Geometry: final body of the model. Coordinates: model frame, mm. A direction names the side the tool comes from. Coordinates: 2 decimals unless noted, no trailing zeros. Write each loop counter-clockwise with the first axis right and the second up, starting at its lowest first coordinate (ties: lowest second). Pieces come first, ordered by that corner, then holes. Notation, with made-up numbers: (-22, 35) -> (-17, 35) arc R36 ccw to (-17, 72) -> close; hole circle Ø6 at (-17, 72.5). An arc over 180 degrees is marked (long way). Answer as a JSON object with one key per item and string values. Group by question number.
```python
from build123d import *

# Parameters (mm, degrees)
SKETCH1_R             = 3
BOSS_EXTRUDE1_DEPTH   = 25
FILLET2_R             = 2
CUT_EXTRUDE1_DEPTH    = 26
M5_TAPPED_HOLE1_D     = 4.2
M5_TAPPED_HOLE1_DEPTH = 22.4
M5_TAPPED_HOLE1_TIP   = 1.2618073
M5_TAPPED_HOLE2_D     = 4.2
M5_TAPPED_HOLE2_DEPTH = 22.4
M5_TAPPED_HOLE2_TIP   = 1.2618073
M4_TAPPED_HOLE1_D     = 3.3
M4_TAPPED_HOLE1_DEPTH = 10.1
M4_TAPPED_HOLE1_TIP   = 0.991420021
CHAMFER1_SIZE         = 1


with BuildPart() as part:
    # Sketch1 → Boss-Extrude1 (new body)
    with BuildSketch(Plane(origin=(0, 0, 0), x_dir=(0, 0, -1), z_dir=(1, 0, 0))):
        with BuildLine():
            Line((-33.809460939, 72.504622963), (-30.428514845, 65.254160667))
            ThreePointArc((-30.428514845, 65.254160667), (-17.004346403, 64.269330845), (-4.58110934, 59.088465181))
            Line((-4.58110934, 59.088465181), (10.41889066, 59.088465181))
            Line((10.41889066, 59.088465181), (13.891854213, 78.784620241))
            ThreePointArc((13.891854213, 78.784620241), (-10.442095378, 79.31558891), (-33.809460939, 72.504622963))
        make_face()
        with Locations((0, 70)):
            Circle(SKETCH1_R, mode=Mode.SUBTRACT)
    extrude(amount=BOSS_EXTRUDE1_DEPTH)

    # Fillet2
    fillet2_edges = [part.edges().sort_by_distance(p)[0] for p in [
        (12.5, 59.088465181, 4.58110934),
        (12.5, 65.254160667, 30.428514845),
        (12.5, 72.504622963, 33.809460939),
        (12.5, 78.784620241, -13.891854213),
        (12.5, 59.088465181, -10.41889066),
    ]]
    fillet(fillet2_edges, radius=FILLET2_R)

    # Sketch3 → Cut-Extrude1 (cut, through all)
    with BuildSketch(Plane(origin=(25, 0, 0), x_dir=(0, 0, -1), z_dir=(1, 0, 0))):
        Polygon((-23.953386268, 80.509473559), (-18.081663619, 82.028004286), (-17.080143603, 78.155413725), (-22.951866252, 76.636882997), align=None)
        Polygon((3.776986852, 89.910790074), (11.540104609, 89.163286855), (11.540104609, 79.163286855), (3.776986852, 79.910790074), align=None)
    extrude(amount=-CUT_EXTRUDE1_DEPTH, mode=Mode.SUBTRACT)

    # M5 Tapped Hole1
    with Locations(Plane(origin=(0, 77.396148361, 20.016004928), x_dir=(1, 0, 0), z_dir=(0, 0.96814764, 0.250380004))):
        with Locations((12.5, 0)):
            Hole(M5_TAPPED_HOLE1_D / 2, depth=M5_TAPPED_HOLE1_DEPTH)
            with Locations((0, 0, -(M5_TAPPED_HOLE1_DEPTH + M5_TAPPED_HOLE1_TIP / 2))):  # 118° drill point
                Cone(0, M5_TAPPED_HOLE1_D / 2, M5_TAPPED_HOLE1_TIP, mode=Mode.SUBTRACT)

    # M5 Tapped Hole2
    with Locations(Plane(origin=(0, 79.537038465, -7.65854573), x_dir=(1, 0, 0), z_dir=(0, 0.995396198, -0.095845753))):
        with Locations((12.5, 0)):
            Hole(M5_TAPPED_HOLE2_D / 2, depth=M5_TAPPED_HOLE2_DEPTH)
            with Locations((0, 0, -(M5_TAPPED_HOLE2_DEPTH + M5_TAPPED_HOLE2_TIP / 2))):  # 118° drill point
                Cone(0, M5_TAPPED_HOLE2_D / 2, M5_TAPPED_HOLE2_TIP, mode=Mode.SUBTRACT)

    # M4 Tapped Hole1
    with Locations(Plane(origin=(0, 59.088465181, 0), x_dir=(-1, 0, 0), z_dir=(0, -1, 0))):
        with Locations((-6.5, 0), (-18.5, 0)):
            Hole(M4_TAPPED_HOLE1_D / 2, depth=M4_TAPPED_HOLE1_DEPTH)
            with Locations((0, 0, -(M4_TAPPED_HOLE1_DEPTH + M4_TAPPED_HOLE1_TIP / 2))):  # 118° drill point
                Cone(0, M4_TAPPED_HOLE1_D / 2, M4_TAPPED_HOLE1_TIP, mode=Mode.SUBTRACT)

    # Chamfer1
    chamfer1_edges = [part.edges().sort_by_distance(p)[0] for p in [
        (25, 70, 3),
        (0, 70, 3),
    ]]
    chamfer(chamfer1_edges, length=CHAMFER1_SIZE)


solid = part.part
```
Item 1: Section D-D on x = 18.5. Output: boundary loops of the cut face in (y, z), then the cut area to 3 significant figures.
Item 2: Contact query for flat-ended pins moving along their axis: pin 1 (2 mm diameter, centred on x = 11, z = 25.5, fed in from -Y); pin 2 (5 mm diameter, centred on y = 70.5, z = 1, fed in from +X); pin 3 (12 mm diameter, centred on x = 16, z = 18, fed in from +Y); pin 4 (3.5 mm diameter, centred on y = 70, z = 0, fed in from +X). Output: stop coordinate, or through.
Item 3: Mould query, pull axis X, two halves, no side actions, for faces 3 (the flat face through (25, 70, 5)), 4 (the cylindrical face through (12.7, 78.3, -13.2)), 5 (the cylindrical face through (14.6, 69, -6.7)). Classes: +X half, -X half, draft (parallel to the pull), parting line (faces both ways), or undercut.
Item 4: Set-up query: faces 1 (the cylindrical face through (16.85, 63.35, -0.07)), 2 (the cylindrical face through (12.675, 59.164, 4.561)). Return all of +Z, -Z, +X, -X, +Y, -Y with unobstructed straight access to the full face (end or side cutting, diameter ignored); none if empty.
Item 5: Section A-A on z = 0. Output: boundary loops of the cut face in (x, y).
Item 6: Section B-B on x = 22.75. Output: boundary loops of the cut face in (y, z), then the cut area to 3 significant figures.
Item 7: Ray query, L1, parallel to X at y = 77.5, z = -8; L2, parallel to Z at x = 18.5, y = 61.25; L3, parallel to Z at x = 8, y = 74. Return the intervals inside material, ascending. Write a range as [from, to].
Item 8: Section C-C on y = 71.75. Give the number of separate pieces and of enclosed holes in the cut face, then the cut area to 3 significant figures.
Answer sheet:
{
 "1": {"outline": "(59.09, -8.74) arc R2 ccw to (60.74, -10.71) -> (76.79, -13.54) arc R2 ccw to (79.11, -11.87) arc R80 ccw to (79.16, -11.54) -> (79.91, -3.78) arc R80 ccw to (78.16, 17.08) -> (76.64, 22.95) arc R80 ccw to (73.35, 31.94) arc R2 ccw to (70.67, 32.95) -> (66.5, 31.01) arc R2 ccw to (65.35, 29.09) arc R42 cw to (59.38, 5.05) arc R2 ccw to (59.09, 4.02) -> (59.09, 1.65) -> (67.49, 1.65) arc R3 cw (long way) to (67.49, -1.65) -> (59.09, -1.65) -> close", "area": "665 mm^2"},
 "2": {"pin 1": "stops at y = 65.36", "pin 2": "stops at x = 24.62", "pin 3": "stops at y = 79.09", "pin 4": "passes through"},
 "3": {"face 3": "+X half", "face 4": "draft", "face 5": "undercut"},
 "4": {"face 1": "-Y", "face 2": "+Z, +X, -X, -Y"},
 "5": {"outline": "(0, 59.09) -> (4.85, 59.09) -> (4.85, 67) -> (1, 67) -> (0, 66) -> close; (0, 74) -> (1, 73) -> (24, 73) -> (25, 74) -> (25, 80) -> (0, 80) -> close; (8.15, 59.09) -> (16.85, 59.09) -> (16.85, 67) -> (8.15, 67) -> close; (20.15, 59.09) -> (25, 59.09) -> (25, 66) -> (24, 67) -> (20.15, 67) -> close"},
 "6": {"outline": "(59.09, -8.74) arc R2 ccw to (60.74, -10.71) -> (76.79, -13.54) arc R2 ccw to (79.11, -11.87) arc R80 ccw to (79.16, -11.54) -> (79.91, -3.78) arc R80 ccw to (78.16, 17.08) -> (76.64, 22.95) arc R80 ccw to (73.35, 31.94) arc R2 ccw to (70.67, 32.95) -> (66.5, 31.01) arc R2 ccw to (65.35, 29.09) arc R42 cw to (59.38, 5.05) arc R2 ccw to (59.09, 4.02) -> close; hole circle Ø6 at (70, 0)", "area": "692 mm^2"},
 "7": {"L1": "x = [0, 10.47], [14.53, 25]", "L2": "z = [-10.8, -1.65], [1.65, 8.51]", "L3": "z = [-13.05, 30.4]"},
 "8": {"separate pieces": "2", "enclosed holes": "2", "area": "992 mm^2"}
}
